from build123d import *

# Parameters (mm, degrees)
SKETCH5_R                = 4.5
BOSS_EXTRUDE2_DEPTH      = 17
SKETCH6_R                = 3.475
CUT_EXTRUDE2_DEPTH       = 9
SKETCH7_R                = 3
CUT_EXTRUDE3_DEPTH       = 9
SKETCH8_W                = 5.3
SKETCH8_H                = 4.2
BOSS_EXTRUDE3_DEPTH      = 18
SKETCH9_W                = 3.3
SKETCH9_H                = 2.2
CUT_EXTRUDE7_DEPTH       = 20
SKETCH22_W               = 2
SKETCH22_H               = 4.219602282
CUT_EXTRUDE17_DEPTH      = 10
SKETCH23_W               = 15.323048642
SKETCH23_H               = 5.208319784
CUT_EXTRUDE18_DEPTH      = 7
SKETCH24_W               = 2
SKETCH24_H               = 5.427023282
CUT_EXTRUDE19_DEPTH      = 18
CUT_EXTRUDE19_DEPTH_BACK = 1
SKETCH26_R               = 3.475
CUT_EXTRUDE21_DEPTH      = 7


with BuildPart() as part:
    # Sketch5 → Boss-Extrude2 (new body)
    with BuildSketch(Plane(origin=(0, 0, 0), x_dir=(1, 0, 0), z_dir=(0, 1, 0))):
        Circle(SKETCH5_R)
    extrude(amount=BOSS_EXTRUDE2_DEPTH)

    # Sketch6 → Cut-Extrude2 (cut)
    with BuildSketch(Plane(origin=(0, 17, 0), x_dir=(1, 0, 0), z_dir=(0, 1, 0))):
        Circle(SKETCH6_R)
    extrude(amount=-CUT_EXTRUDE2_DEPTH, mode=Mode.SUBTRACT)

    # Sketch7 → Cut-Extrude3 (cut, through all)
    with BuildSketch(Plane(origin=(0, 8, 0), x_dir=(1, 0, 0), z_dir=(0, 1, 0))):
        Circle(SKETCH7_R)
    extrude(amount=-CUT_EXTRUDE3_DEPTH, mode=Mode.SUBTRACT)

    # Sketch8 → Boss-Extrude3 (add)
    with BuildSketch(Plane.XY.offset(3)):
        with Locations((0, 14.9)):
            Rectangle(SKETCH8_W, SKETCH8_H)
    extrude(amount=BOSS_EXTRUDE3_DEPTH)

    # Sketch9 → Cut-Extrude7 (cut)
    with BuildSketch(Plane.XY.offset(21)):
        with Locations((0, 14.9)):
            Rectangle(SKETCH9_W, SKETCH9_H)
    extrude(amount=-CUT_EXTRUDE7_DEPTH, mode=Mode.SUBTRACT)

    # Sketch22 → Cut-Extrude17 (cut)
    with BuildSketch(Plane(origin=(0, 0, 0), x_dir=(1, 0, 0), z_dir=(0, 1, 0))):
        with Locations((0, -4.5)):
            Rectangle(SKETCH22_W, SKETCH22_H)
    extrude(amount=CUT_EXTRUDE17_DEPTH, mode=Mode.SUBTRACT)

    # Sketch23 → Cut-Extrude18 (cut)
    with BuildSketch(Plane(origin=(0, 0, 0), x_dir=(1, 0, 0), z_dir=(0, 1, 0))):
        with Locations((-0.238082605, -2.604159892)):
            Rectangle(SKETCH23_W, SKETCH23_H)
    extrude(amount=CUT_EXTRUDE18_DEPTH, mode=Mode.SUBTRACT)

    # Sketch24 → Cut-Extrude19 (cut, two sides)
    with BuildSketch(Plane(origin=(0, 0, 0), x_dir=(1, 0, 0), z_dir=(0, 1, 0))) as cut_extrude19_sk:
        with Locations((0, 4.5)):
            Rectangle(SKETCH24_W, SKETCH24_H)
    extrude(amount=CUT_EXTRUDE19_DEPTH, mode=Mode.SUBTRACT)
    extrude(cut_extrude19_sk.sketch, amount=-CUT_EXTRUDE19_DEPTH_BACK, mode=Mode.SUBTRACT)

    # Sketch26 → Cut-Extrude21 (cut)
    with BuildSketch(Plane(origin=(0, 17, 0), x_dir=(1, 0, 0), z_dir=(0, 1, 0))):
        Circle(SKETCH26_R)
    extrude(amount=-CUT_EXTRUDE21_DEPTH, mode=Mode.SUBTRACT)


solid = part.part
Read the model definition and answer for the solid it produces. Units are mm, in the model's axes. A direction names the side the tool comes from. Round coordinates to 2 decimals unless told otherwise and drop trailing zeros. Order: outer loops, then holes, each group sorted by start corner. A loop starts at its lowest first (then second) coordinate and runs counter-clockwise, first axis right, second up. Notation, with made-up numbers: (59, 65) - (76, 65) arc R17 cw to (76, 73) - close; hole circle Ø6 at (88.25, 62). An arc over 180 degrees is marked (long way). Use one line per item in the form item = value. Start each with the question number.
(1) The part is cut by section A-A (y = 14.5). Give the vertices of the cut face in (x, z) (3 decimals).
(2) Find the intervals of material crossed by line 1 along Y through (x, z) = (-1.5, 16); line 2 along X through (y, z) = (12.5, 0) (3 decimals); line 3 along X through (y, z) = (14, 10), in increasing order. Write a range as from..to.
(3) Determine the mould class of faces 6 (the face through (-3, 7, 2)), 7 (the face through (0, 13.8, 12)), 8 (the face through (-3, 8, -1)) for opening direction Y: +Y half, -Y half, draft (parallel to the pull), parting line (faces both ways), or undercut.
(4) The part is cut by section C-C (z = 13). Give the vertices of the cut face in (x, y).
(5) The part is cut by section D-D (y = 7.5). Give the vertices of the cut face in (x, z).
(6) Flat-ended cylindrical pins translate along their axes: pin 1 Ø1.1 at (y, z) = (14.5, 14.5) entering from -X; pin 2 Ø1.1 at (y, z) = (15, 9.5) entering from +X; pin 3 Ø1.2 at (x, y) = (-3.5, 5) entering from +Z; pin 4 Ø10 at (y, z) = (5, 14.5) entering from +X. Find the tip coordinate at first contact, or state that the pin passes through.
(7) For faces 1 (the face through (1.65, 15, 12)), 2 (the face through (-0.139, 12.563, 3.472)), 3 (the face through (-4, 3, 0)), 4 (the face through (-1, 8, -4)), 5 (the face through (-2.535, 4.056, -1.605)), determine the directions among +Z, -Z, +X, -X, +Y, -Y from which every point of the face is accessible in a straight line to the end or side of a thin tool.
(8) The part is cut by section B-B (x = 0). Give the vertices of the cut face in (y, z) (3 decimals).
Checked values:
q1.outline = (-2.65, 3.637) arc R4.5 ccw to (-1, -4.387) - (-1, -3.328) arc R3.475 cw to (-1.65, 3.058) - (-1.65, 21) - (-2.65, 21) - close; (1, -4.387) arc R4.5 ccw to (2.65, 3.637) - (2.65, 21) - (1.65, 21) - (1.65, 3.058) arc R3.475 cw to (1, -3.328) - close
q2.line_1 = 12.8..13.8, 16..17
q2.line_2 = -4.5..-3.475, 3.475..4.5
q2.line_3 = -2.65..-1.65, 1.65..2.65
q3.face_6 = -Y half
q3.face_7 = undercut
q3.face_8 = +Y half
q4.outline = (-2.65, 12.8) - (2.65, 12.8) - (2.65, 17) - (-2.65, 17) - close; hole (-1.65, 13.8) - (1.65, 13.8) - (1.65, 16) - (-1.65, 16) - close
q5.outline = (-1, -4.39) - (-1, -2.83) arc R3 cw to (-1, 2.83) - (-1, 4.39) arc R4.5 ccw to start; (1, -4.39) arc R4.5 ccw to (1, 4.39) - (1, 2.83) arc R3 cw to (1, -2.83) - close
q6.pin_1 = -2.65
q6.pin_2 = 2.65
q6.pin_3 = 0
q6.pin_4 = through
q7.face_1 = +Z
q7.face_2 = +Y
q7.face_3 = +Z, +X, -X, -Y
q7.face_4 = -Z, +Y, -Y
q7.face_5 = +Y, -Y
q8.outline = (10, 3.475) - (13.8, 3.475) - (13.8, 21) - (12.8, 21) - (12.8, 4.5) - (10, 4.5) - close; (16, 3.475) - (17, 3.475) - (17, 21) - (16, 21) - close
